from build123d import *

# Parameters (mm, degrees)
F0_R      = 6
F1_DEPTH  = 4
F2_R      = 6
F2_R_2    = 4.6
F3_DEPTH  = 20
F6_DEPTH  = 25
F9_DEPTH  = 0.3
F11_DEPTH = 10


with BuildPart() as f1:
    # F0 (on Top) → F1 (new body)
    with BuildSketch(Plane.XY):
        Circle(F0_R)
    extrude(amount=F1_DEPTH)

    # F2 (on face) → F3 (join)
    with BuildSketch(Plane.XY.offset(4)):
        Circle(F2_R)
        Circle(F2_R_2, mode=Mode.SUBTRACT)
    extrude(amount=F3_DEPTH)

    # F5 (on offset) → F6 (cut)
    with BuildSketch(Plane.XZ.offset(10)):
        with BuildLine():
            ThreePointArc((-2.6, 3.75), (-2.8196699141, 4.2803300859), (-3.35, 4.5))
            Line((-3.35, 4.5), (-3.35, 3))
            ThreePointArc((-3.35, 3), (-2.8196699141, 3.2196699141), (-2.6, 3.75))
        make_face()
        with BuildLine():
            Line((3.35, 4.5), (-3.35, 4.5))
            ThreePointArc((-3.35, 4.5), (-2.8196699141, 4.2803300859), (-2.6, 3.75))
            ThreePointArc((-2.6, 3.75), (-2.8196699141, 3.2196699141), (-3.35, 3))
            Line((-3.35, 3), (3.35, 3))
            ThreePointArc((3.35, 3), (2.6, 3.75), (3.35, 4.5))
        make_face()
        with BuildLine():
            Line((-3.35, 3), (-3.35, 4.5))
            ThreePointArc((-3.35, 4.5), (-4.1, 3.75), (-3.35, 3))
        make_face()
        with BuildLine():
            ThreePointArc((4.1, 3.75), (3.8803300859, 4.2803300859), (3.35, 4.5))
            Line((3.35, 4.5), (3.35, 3))
            ThreePointArc((3.35, 3), (3.8803300859, 3.2196699141), (4.1, 3.75))
        make_face()
        with BuildLine():
            Line((3.35, 3), (3.35, 4.5))
            ThreePointArc((3.35, 4.5), (2.6, 3.75), (3.35, 3))
        make_face()
    extrude(amount=-F6_DEPTH, mode=Mode.SUBTRACT)

    # F8 (on offset) → F9 (join)
    with BuildSketch(Plane(origin=(0, 0, 10), x_dir=(1, 0, 0), z_dir=(0, 0, -1))):
        with BuildLine():
            ThreePointArc((-3.7672105065, -2.175), (-4.35, 0), (-3.7672105065, 2.175))
            Line((-3.7672105065, 2.175), (-3.9837168574, 2.3))
            ThreePointArc((-3.9837168574, 2.3), (-4.6, 0), (-3.9837168574, -2.3))
            Line((-3.9837168574, -2.3), (-3.7672105065, -2.175))
        make_face()
        with BuildLine():
            Line((3.7672105065, -2.175), (3.9837168574, -2.3))
            ThreePointArc((3.9837168574, -2.3), (4.6, 0), (3.9837168574, 2.3))
            Line((3.9837168574, 2.3), (3.7672105065, 2.175))
            ThreePointArc((3.7672105065, 2.175), (4.35, 0), (3.7672105065, -2.175))
        make_face()
    extrude(amount=-F9_DEPTH)

    # F10 (on offset) → F11 (cut)
    with BuildSketch(Plane.XZ.offset(10)):
        with BuildLine():
            ThreePointArc((-2.6, 9.05), (-2.8196699141, 9.5803300859), (-3.35, 9.8))
            Line((-3.35, 9.8), (-3.35, 8.3))
            ThreePointArc((-3.35, 8.3), (-2.8196699141, 8.5196699141), (-2.6, 9.05))
        make_face()
        with BuildLine():
            Line((3.35, 9.8), (-3.35, 9.8))
            ThreePointArc((-3.35, 9.8), (-2.8196699141, 9.5803300859), (-2.6, 9.05))
            ThreePointArc((-2.6, 9.05), (-2.8196699141, 8.5196699141), (-3.35, 8.3))
            Line((-3.35, 8.3), (3.35, 8.3))
            ThreePointArc((3.35, 8.3), (2.6, 9.05), (3.35, 9.8))
        make_face()
        with BuildLine():
            Line((-3.35, 8.3), (-3.35, 9.8))
            ThreePointArc((-3.35, 9.8), (-4.1, 9.05), (-3.35, 8.3))
        make_face()
        with BuildLine():
            ThreePointArc((4.1, 9.05), (3.8803300859, 9.5803300859), (3.35, 9.8))
            Line((3.35, 9.8), (3.35, 8.3))
            ThreePointArc((3.35, 8.3), (3.8803300859, 8.5196699141), (4.1, 9.05))
        make_face()
        with BuildLine():
            Line((3.35, 8.3), (3.35, 9.8))
            ThreePointArc((3.35, 9.8), (2.6, 9.05), (3.35, 8.3))
        make_face()
    extrude(amount=-F11_DEPTH, mode=Mode.SUBTRACT)


solid = f1.part
Geometry: final body of the model. Coordinates: model frame, mm. A direction names the side the tool comes from. Round coordinates to 2 decimals unless told otherwise and drop trailing zeros. Loops run counter-clockwise (first coordinate to the right, second up) from the corner with the lowest first, then second, coordinate; pieces in that order, holes last.
Q1. Section D-D on z = 2.25. Return loops of the section in (x, y).
Q2. Material intervals for L1, parallel to Z at x = 2.5, y = -5.25; L2, parallel to Y at x = 0, z = 12.75; L3, parallel to Z at x = 0.5, y = 5, sorted ascending.
Q3. Access query for faces 4 (the flat face through (0, -5, 8.3)), 5 (the flat face through (3, -4, 24)), 6 (the flat face through (0, 5, 4.5)). Directions: +Z, -Z, +X, -X, +Y, -Y. A direction counts if a zero-diameter tool reaches every point of the face in a straight line with its end or side. Return the directions, or none.
Q4. Pin query (flat end, axial travel): P1, Ø2.5, axis at x = 1.5, y = -5, coming from the -Z side; P2, Ø5, axis at y = 3, z = 14, coming from the +X side; P3, Ø2, axis at x = 0.5, y = 0, coming from the +Z side; P4, Ø5, axis at x = -4, z = 20, coming from the -Y side. Return the tip coordinate at first contact, or that it passes through.
Q5. Pull-direction query (X, two-part tool) for faces 1 (the flat face through (0, -5, 9.8)), 2 (the cylindrical face through (-0.78, 5.95, 11.83)), 3 (the flat face through (0, 0, 0)); classes: released by +X, released by -X, zero draft, split by the parting line, or undercut.
Q6. Section A-A on x = 0. Return loops of the section in (y, z), plus the area to 3 significant figures.
Q7. Section B-B on y = 0. Return loops of the section in (x, z), plus the area to 3 significant figures.
Q8. Section C-C on z = 15. Return loops of the section in (x, y).
Evaluation:
1. outline: circle Ø12 at (0, 0)
2. L1: z = 0 to 3, 4.5 to 8.3, 9.8 to 24
2. L2: y = -6 to -4.6, 4.6 to 6
2. L3: z = 0 to 3, 4.5 to 24
3. face 4: -Y
3. face 5: +Z, +X, -X, +Y, -Y
3. face 6: +Y, -Y
4. P1: stops at z = 0
4. P2: stops at x = 5.98
4. P3: stops at z = 3
4. P4: stops at y = -5.81
5. face 1: undercut
5. face 2: split by the parting line
5. face 3: zero draft
6. outline: (-6, 0) - (6, 0) - (6, 3) - (-6, 3) - close; (-6, 4.5) - (-4.6, 4.5) - (-4.6, 8.3) - (-6, 8.3) - close; (-6, 9.8) - (-4.6, 9.8) - (-4.6, 24) - (-6, 24) - close; (4.6, 4.5) - (6, 4.5) - (6, 24) - (4.6, 24) - close
6. area: 88.5 mm2
7. outline: (-6, 0) - (6, 0) - (6, 24) - (4.6, 24) - (4.6, 10.3) - (4.35, 10.3) - (4.35, 10) - (4.6, 10) - (4.6, 4) - (4.06, 4) arc R0.75 cw to (3.35, 3) - (-3.35, 3) arc R0.75 cw to (-4.06, 4) - (-4.6, 4) - (-4.6, 10) - (-4.35, 10) - (-4.35, 10.3) - (-4.6, 10.3) - (-4.6, 24) - (-6, 24) - close
7. area: 96.2 mm2
8. outline: circle Ø12 at (0, 0); hole circle Ø9.2 at (0, 0)
